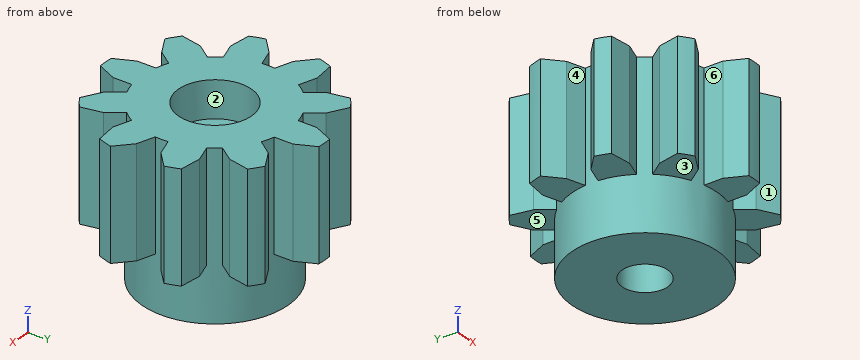
from build123d import *

# Parameters (mm, degrees)
SKETCH_1_W                   = 4
SKETCH_1_H                   = 9
EXTRUDE_1_DEPTH              = 6
EXTRUDE_2_DEPTH              = 6
EXTRUDE_3_DEPTH              = 6
EXTRUDE_4_DEPTH              = 6
EXTRUDE_5_DEPTH              = 6
EXTRUDE_6_DEPTH              = 6
EXTRUDE_7_DEPTH              = 6
EXTRUDE_8_DEPTH              = 6
EXTRUDE_9_DEPTH              = 6
EXTRUDE_10_DEPTH             = 6
HOLE_WIZARD_M2_1_D           = 2.5
HOLE_WIZARD_M2_1_CBORE_D     = 4
HOLE_WIZARD_M2_1_CBORE_DEPTH = 2


with BuildPart() as part:
    # 草图1 → 旋转1 (revolve)
    with BuildSketch(Plane.XZ, mode=Mode.PRIVATE) as revolve_1_sk:
        with Locations((2, 1.5)):
            Rectangle(SKETCH_1_W, SKETCH_1_H)
    revolve(revolve_1_sk.sketch.rotate(Axis((0, 0, 6), (0, 0, -1)), 180), axis=Axis((0, 0, 6), (0, 0, -1)))

    # 草图2 → 凸台-拉伸1 (add)
    with BuildSketch(Plane.XY.offset(6)):
        with BuildLine():
            Line((3.984468068, 0.352156525), (4.955233641, 0.66757738))
            Line((4.955233641, 0.66757738), (5.818800307, 1.463408004))
            ThreePointArc((5.818800307, 1.463408004), (5.706339098, 1.854101966), (5.567677978, 2.236283062))
            Line((5.567677978, 2.236283062), (4.401260366, 2.372531811))
            Line((4.401260366, 2.372531811), (3.430494792, 2.057110955))
            ThreePointArc((3.430494792, 2.057110955), (3.804226065, 1.236067977), (3.984468068, 0.352156525))
        make_face()
    extrude(amount=-EXTRUDE_1_DEPTH)

    # 草图3 → 凸台-拉伸2 (add)
    with BuildSketch(Plane.XY.offset(6)):
        with BuildLine():
            Line((3.016509969, 2.626912182), (3.616476088, 3.452694702))
            Line((3.616476088, 3.452694702), (3.847338693, 4.604126951))
            ThreePointArc((3.847338693, 4.604126951), (3.526711514, 4.854101966), (3.1898919, 5.081790006))
            Line((3.1898919, 5.081790006), (2.166155224, 4.506414489))
            Line((2.166155224, 4.506414489), (1.566189104, 3.680631969))
            ThreePointArc((1.566189104, 3.680631969), (2.351141009, 3.236067977), (3.016509969, 2.626912182))
        make_face()
    extrude(amount=-EXTRUDE_2_DEPTH)

    # 草图4 → 凸台-拉伸3 (add)
    with BuildSketch(Plane.XY.offset(6)):
        with BuildLine():
            Line((0.896347589, 3.898276671), (0.896347589, 4.919))
            Line((0.896347589, 4.919), (0.406324464, 5.986225892))
            ThreePointArc((0.406324464, 5.986225892), (0, 6), (-0.406324464, 5.986225892))
            Line((-0.406324464, 5.986225892), (-0.896347589, 4.919))
            Line((-0.896347589, 4.919), (-0.896347589, 3.898276671))
            ThreePointArc((-0.896347589, 3.898276671), (0, 4), (0.896347589, 3.898276671))
        make_face()
    extrude(amount=-EXTRUDE_3_DEPTH)

    # 草图5 → 凸台-拉伸4 (add)
    with BuildSketch(Plane.XY.offset(6)):
        with BuildLine():
            Line((-1.566189104, 3.680631969), (-2.166155224, 4.506414489))
            Line((-2.166155224, 4.506414489), (-3.1898919, 5.081790006))
            ThreePointArc((-3.1898919, 5.081790006), (-3.526711514, 4.854101966), (-3.847338693, 4.604126951))
            Line((-3.847338693, 4.604126951), (-3.616476088, 3.452694702))
            Line((-3.616476088, 3.452694702), (-3.016509969, 2.626912182))
            ThreePointArc((-3.016509969, 2.626912182), (-2.351141009, 3.236067977), (-1.566189104, 3.680631969))
        make_face()
    extrude(amount=-EXTRUDE_4_DEPTH)

    # 草图6 → 凸台-拉伸5 (add)
    with BuildSketch(Plane.XY.offset(6)):
        with BuildLine():
            Line((-3.430494792, 2.057110955), (-4.401260366, 2.372531811))
            Line((-4.401260366, 2.372531811), (-5.567677978, 2.236283062))
            ThreePointArc((-5.567677978, 2.236283062), (-5.706339098, 1.854101966), (-5.818800307, 1.463408004))
            Line((-5.818800307, 1.463408004), (-4.955233641, 0.66757738))
            Line((-4.955233641, 0.66757738), (-3.984468068, 0.352156525))
            ThreePointArc((-3.984468068, 0.352156525), (-3.804226065, 1.236067977), (-3.430494792, 2.057110955))
        make_face()
    extrude(amount=-EXTRUDE_5_DEPTH)

    # 草图7 → 凸台-拉伸6 (add)
    with BuildSketch(Plane.XY.offset(6)):
        with BuildLine():
            Line((-3.984468068, -0.352156525), (-4.955233641, -0.66757738))
            Line((-4.955233641, -0.66757738), (-5.818800307, -1.463408004))
            ThreePointArc((-5.818800307, -1.463408004), (-5.706339098, -1.854101966), (-5.567677978, -2.236283062))
            Line((-5.567677978, -2.236283062), (-4.401260366, -2.372531811))
            Line((-4.401260366, -2.372531811), (-3.430494792, -2.057110955))
            ThreePointArc((-3.430494792, -2.057110955), (-3.804226065, -1.236067977), (-3.984468068, -0.352156525))
        make_face()
    extrude(amount=-EXTRUDE_6_DEPTH)

    # 草图8 → 凸台-拉伸7 (add)
    with BuildSketch(Plane.XY.offset(6)):
        with BuildLine():
            Line((-3.016509969, -2.626912182), (-3.616476088, -3.452694702))
            Line((-3.616476088, -3.452694702), (-3.847338693, -4.604126951))
            ThreePointArc((-3.847338693, -4.604126951), (-3.526711514, -4.854101966), (-3.1898919, -5.081790006))
            Line((-3.1898919, -5.081790006), (-2.166155224, -4.506414489))
            Line((-2.166155224, -4.506414489), (-1.566189104, -3.680631969))
            ThreePointArc((-1.566189104, -3.680631969), (-2.351141009, -3.236067977), (-3.016509969, -2.626912182))
        make_face()
    extrude(amount=-EXTRUDE_7_DEPTH)

    # 草图9 → 凸台-拉伸8 (add)
    with BuildSketch(Plane.XY.offset(6)):
        with BuildLine():
            Line((-0.896347589, -3.898276671), (-0.896347589, -4.919))
            Line((-0.896347589, -4.919), (-0.406324464, -5.986225892))
            ThreePointArc((-0.406324464, -5.986225892), (0, -6), (0.406324464, -5.986225892))
            Line((0.406324464, -5.986225892), (0.896347589, -4.919))
            Line((0.896347589, -4.919), (0.896347589, -3.898276671))
            ThreePointArc((0.896347589, -3.898276671), (0, -4), (-0.896347589, -3.898276671))
        make_face()
    extrude(amount=-EXTRUDE_8_DEPTH)

    # 草图10 → 凸台-拉伸9 (add)
    with BuildSketch(Plane.XY.offset(6)):
        with BuildLine():
            Line((1.566189104, -3.680631969), (2.166155224, -4.506414489))
            Line((2.166155224, -4.506414489), (3.1898919, -5.081790006))
            ThreePointArc((3.1898919, -5.081790006), (3.526711514, -4.854101966), (3.847338693, -4.604126951))
            Line((3.847338693, -4.604126951), (3.616476088, -3.452694702))
            Line((3.616476088, -3.452694702), (3.016509969, -2.626912182))
            ThreePointArc((3.016509969, -2.626912182), (2.351141009, -3.236067977), (1.566189104, -3.680631969))
        make_face()
    extrude(amount=-EXTRUDE_9_DEPTH)

    # 草图11 → 凸台-拉伸10 (add)
    with BuildSketch(Plane.XY.offset(6)):
        with BuildLine():
            Line((3.430494792, -2.057110955), (4.401260366, -2.372531811))
            Line((4.401260366, -2.372531811), (5.567677978, -2.236283062))
            ThreePointArc((5.567677978, -2.236283062), (5.706339098, -1.854101966), (5.818800307, -1.463408004))
            Line((5.818800307, -1.463408004), (4.955233641, -0.66757738))
            Line((4.955233641, -0.66757738), (3.984468068, -0.352156525))
            ThreePointArc((3.984468068, -0.352156525), (3.804226065, -1.236067977), (3.430494792, -2.057110955))
        make_face()
    extrude(amount=-EXTRUDE_10_DEPTH)

    # M2 六角头机械螺钉的柱形沉头孔1 (through all)
    with Locations(Plane.XY.offset(6)):
        with Locations((0, 0)):
            CounterBoreHole(HOLE_WIZARD_M2_1_D / 2, HOLE_WIZARD_M2_1_CBORE_D / 2, HOLE_WIZARD_M2_1_CBORE_DEPTH)


solid = part.part
The model under review builds one solid part; all positions refer to its coordinate system, in mm. Face numbers are marked on the shaded views. A direction names the side the tool comes from. Round coordinates to 2 decimals unless told otherwise and drop trailing zeros. Write each loop counter-clockwise with the first axis right and the second up, starting at its lowest first coordinate (ties: lowest second). Pieces come first, ordered by that corner, then holes. Notation, with made-up numbers: (19.5, 11.25) - (77.5, 11.25) arc R14 ccw to (77.5, 23.25) - close; hole circle Ø1 at (78.5, 5.5). An arc over 180 degrees is marked (long way). One line per item, written item: value. Start each with the question number.
1. To check wall thickness, follow L1, parallel to X at y = 5, z = 0.25; L2, parallel to Y at x = 0, z = 1.5; L3, parallel to Y at x = 0, z = 5. State the ranges of each line that lie inside material, in increasing order. Write a range as from..to.
2. Clearance check with flat-ended pins moving along their axes: P1, Ø1, axis at y = -4.5, z = 0, coming from the +X side; P2, Ø1.8, axis at x = -3, y = 4, coming from the -Z side; P3, Ø3, axis at x = 0, y = 0, coming from the -Z side; P4, Ø1.5, axis at x = 2.5, z = 3.5, coming from the -Y side. State where each tip first meets the part, or that it passes through.
3. Consider section B-B on x = 0. Write out the cut boundary in (y, z).
4. The part is to be moulded in two halves that separate along Y. For the marked faces 1, 2 and 3, say which applies: released by +Y, released by -Y, zero draft, split by the parting line, or undercut.
5. Consider section A-A on y = 0. Write out the cut boundary in (x, z).
6. Consider section C-C on x = -2.5. Write out the cut boundary in (y, z), and give its area (3 significant figures).
7. Machinability: for the marked faces 4, 5 and 6, which of the approach directions +Z, -Z, +X, -X, +Y, -Y give a long, thin tool a straight path to every point of the face, cutting with its end or side? Answer none if there is none.
Checks:
1. L1: x = -3.32..-3.04, -0.86..0.86, 3.04..3.32
1. L2: y = -6..-1.25, 1.25..6
1. L3: y = -6..-2, 2..6
2. P1: stops at x = 3.85
2. P2: stops at z = 0
2. P3: stops at z = -3
2. P4: stops at y = -5.08
3. outline: (-6, 0) - (-4, 0) - (-4, -3) - (-1.25, -3) - (-1.25, 4) - (-2, 4) - (-2, 6) - (-6, 6) - close; (1.25, -3) - (4, -3) - (4, 0) - (6, 0) - (6, 6) - (2, 6) - (2, 4) - (1.25, 4) - close
4. face 1: released by -Y
4. face 2: undercut
4. face 3: zero draft
5. outline: (-4, -3) - (-1.25, -3) - (-1.25, 4) - (-2, 4) - (-2, 6) - (-4, 6) - close; (1.25, -3) - (4, -3) - (4, 6) - (2, 6) - (2, 4) - (1.25, 4) - close
6. outline: (-4.69, 0) - (-3.12, 0) - (-3.12, -3) - (3.12, -3) - (3.12, 0) - (4.69, 0) - (4.69, 6) - (-4.69, 6) - close
6. area: 75.1 mm^2
7. face 4: +Z, -Z, -X
7. face 5: -Z, -X, +Y
7. face 6: +Z, -Z, -Y
